from build123d import *

# Parameters (mm, degrees)
F1_DEPTH = 10


with BuildPart() as f1:
    # F0 (on Top) → F1 (new body)
    with BuildSketch(Plane.XY):
        with BuildLine():
            ThreePointArc((2, 4.582576), (4.894532, -1.021548), (0, -5))
            Line((0, -5), (0, -6.00455))
            Line((0, -6.00455), (5, -6.00455))
            Line((5, -6.00455), (5, -16.00455))
            Line((5, -16.00455), (0, -16.00455))
            Line((0, -16.00455), (0, -17.00455))
            Line((0, -17.00455), (6, -17.002946))
            Line((6, -17.002946), (8.996743, -17.002144))
            Line((8.996743, -17.002144), (8.996987, -16.00455))
            Line((8.996987, -16.00455), (9.259669, -14.657077))
            Line((9.259669, -14.657077), (6, -14.657077))
            Line((6, -14.657077), (6, -13.472727))
            Line((6, -13.472727), (9.490384, -13.473582))
            Line((9.490384, -13.473582), (9.731471, -12.236885))
            Line((9.731471, -12.236885), (6, -12.236885))
            Line((6, -12.236885), (6, -11.00455))
            Line((6, -11.00455), (9.971708, -11.00455))
            Line((9.971708, -11.00455), (10.053972, -9.866621))
            Line((10.053972, -9.866621), (6, -9.863548))
            Line((6, -9.863548), (6, -9.04429))
            Line((6, -9.04429), (10.353642, -9.045355))
            Line((10.353642, -9.045355), (10.554617, -8.01442))
            Line((10.554617, -8.01442), (6, -8.01442))
            Line((6, -8.01442), (6, -6.00455))
            Line((6, -6.00455), (10.946429, -6.00455))
            Line((10.946429, -6.00455), (11.140614, -5.008447))
            Line((11.140614, -5.008447), (6, -5.00455))
            Line((6, -5.00455), (3.316625, -5))
            ThreePointArc((3.316625, -5), (3.879995, -4.57664), (4.389841, -4.090146))
            ThreePointArc((4.389841, -4.090146), (4.809454, -3.587359), (5.171773, -3.041836))
            ThreePointArc((5.171773, -3.041836), (5.483753, -2.434842), (5.724784, -1.796345))
            ThreePointArc((5.724784, -1.796345), (5.863661, -1.271801), (5.954582, -0.736856))
            ThreePointArc((5.954582, -0.736856), (5.999496, -0.077783), (5.971684, 0.582233))
            ThreePointArc((5.971684, 0.582233), (5.902156, 1.079145), (5.791354, 1.56851))
            ThreePointArc((5.791354, 1.56851), (4.789612, 3.61381), (3.097802, 5.138446))
            Line((3.097802, 5.138446), (3.097802, 11.138446))
            Line((3.097802, 11.138446), (2, 11.138446))
            Line((2, 11.138446), (2, 4.582576))
        make_face()
        with BuildLine():
            Line((12.501639, 2.997855), (5.791354, 1.56851))
            ThreePointArc((5.791354, 1.56851), (5.902156, 1.079145), (5.971684, 0.582233))
            Line((5.971684, 0.582233), (12.501639, 1.973166))
            Line((12.501639, 1.973166), (12.501639, 2.997855))
        make_face()
        with BuildLine():
            Line((12.116982, 0), (5.954582, -0.736856))
            ThreePointArc((5.954582, -0.736856), (5.863661, -1.271801), (5.724784, -1.796345))
            Line((5.724784, -1.796345), (11.884799, -1.19102))
            Line((11.884799, -1.19102), (12.116982, 0))
        make_face()
        with BuildLine():
            Line((11.523993, -3.041836), (5.171773, -3.041836))
            ThreePointArc((5.171773, -3.041836), (4.809454, -3.587359), (4.389841, -4.090146))
            Line((4.389841, -4.090146), (11.319631, -4.090146))
            Line((11.319631, -4.090146), (11.523993, -3.041836))
        make_face()
        with BuildLine():
            Line((0, -6.00455), (0, -5))
            ThreePointArc((0, -5), (-4.894532, -1.021548), (-2, 4.582576))
            Line((-2, 4.582576), (-2, 11.138446))
            Line((-2, 11.138446), (-3.097802, 11.138446))
            Line((-3.097802, 11.138446), (-3.097802, 5.138446))
            ThreePointArc((-3.097802, 5.138446), (-4.789612, 3.61381), (-5.791354, 1.56851))
            ThreePointArc((-5.791354, 1.56851), (-5.902156, 1.079145), (-5.971684, 0.582233))
            ThreePointArc((-5.971684, 0.582233), (-5.999496, -0.077783), (-5.954582, -0.736856))
            ThreePointArc((-5.954582, -0.736856), (-5.863661, -1.271801), (-5.724784, -1.796345))
            ThreePointArc((-5.724784, -1.796345), (-5.483753, -2.434842), (-5.171773, -3.041836))
            ThreePointArc((-5.171773, -3.041836), (-4.809454, -3.587359), (-4.389841, -4.090146))
            ThreePointArc((-4.389841, -4.090146), (-3.879995, -4.57664), (-3.316625, -5))
            Line((-3.316625, -5), (-6, -5.00455))
            Line((-6, -5.00455), (-11.140614, -5.008447))
            Line((-11.140614, -5.008447), (-10.946429, -6.00455))
            Line((-10.946429, -6.00455), (-6, -6.00455))
            Line((-6, -6.00455), (-6, -8.01442))
            Line((-6, -8.01442), (-10.554617, -8.01442))
            Line((-10.554617, -8.01442), (-10.353642, -9.045355))
            Line((-10.353642, -9.045355), (-6, -9.04429))
            Line((-6, -9.04429), (-6, -9.863548))
            Line((-6, -9.863548), (-10.053972, -9.866621))
            Line((-10.053972, -9.866621), (-9.971708, -11.00455))
            Line((-9.971708, -11.00455), (-6, -11.00455))
            Line((-6, -11.00455), (-6, -12.236885))
            Line((-6, -12.236885), (-9.731471, -12.236885))
            Line((-9.731471, -12.236885), (-9.490384, -13.473582))
            Line((-9.490384, -13.473582), (-6, -13.472727))
            Line((-6, -13.472727), (-6, -14.657077))
            Line((-6, -14.657077), (-9.259669, -14.657077))
            Line((-9.259669, -14.657077), (-8.996987, -16.00455))
            Line((-8.996987, -16.00455), (-8.996743, -17.002144))
            Line((-8.996743, -17.002144), (-6, -17.002946))
            Line((-6, -17.002946), (0, -17.00455))
            Line((0, -17.00455), (0, -16.00455))
            Line((0, -16.00455), (-5, -16.00455))
            Line((-5, -16.00455), (-5, -6.00455))
            Line((-5, -6.00455), (0, -6.00455))
        make_face()
        with BuildLine():
            ThreePointArc((-5.971684, 0.582233), (-5.902156, 1.079145), (-5.791354, 1.56851))
            Line((-5.791354, 1.56851), (-12.501639, 2.997855))
            Line((-12.501639, 2.997855), (-12.501639, 1.973166))
            Line((-12.501639, 1.973166), (-5.971684, 0.582233))
        make_face()
        with BuildLine():
            ThreePointArc((-5.724784, -1.796345), (-5.863661, -1.271801), (-5.954582, -0.736856))
            Line((-5.954582, -0.736856), (-12.116982, 0))
            Line((-12.116982, 0), (-11.884799, -1.19102))
            Line((-11.884799, -1.19102), (-5.724784, -1.796345))
        make_face()
        with BuildLine():
            ThreePointArc((-4.389841, -4.090146), (-4.809454, -3.587359), (-5.171773, -3.041836))
            Line((-5.171773, -3.041836), (-11.523993, -3.041836))
            Line((-11.523993, -3.041836), (-11.319631, -4.090146))
            Line((-11.319631, -4.090146), (-4.389841, -4.090146))
        make_face()
    extrude(amount=F1_DEPTH)


solid = f1.part
For this review, take the finished solid that the model builds, in its own axes (mm). A direction names the side the tool comes from. Round coordinates to 2 decimals unless told otherwise and drop trailing zeros. Write each loop counter-clockwise with the first axis right and the second up, starting at its lowest first coordinate (ties: lowest second). Pieces come first, ordered by that corner, then holes. Notation, with made-up numbers: M 70,25.25 L 115,25.25 A29 cw 115,54.25 Z; hole C 3,58 d3. An arc over 180 degrees is marked long. Write item = value, one per line. Start each with the question number.
(1) We need section B-B (x = 7). Give the number of separate pieces and of enclosed holes in the cut face, then the cut area to 3 significant figures.
(2) We need section A-A (y = 7.75). Give the boundary of the cut face in (x, z), then the cut area to 3 significant figures.
(3) We need section C-C (y = -15). Give the boundary of the cut face in (x, z).
(4) Clearance check with flat-ended pins moving along their axes: pin 1 Ø4 at (x, z) = (-8, 6.5) entering from +Y (3 decimals); pin 2 Ø3 at (y, z) = (-3, 2.5) entering from +X; pin 3 Ø5 at (y, z) = (8, 7) entering from -X; pin 4 Ø1.5 at (x, y) = (-7.5, -7) entering from -Z. State where each tip first meets the part, or that it passes through.
(5) The part is to be moulded in two halves that separate along X. For faces 4 (the face through (6, -7, 5)), 5 (the face through (2.6, 11.138, 4.9)), 6 (the face through (-6, 0, 5)), say which applies: +X half, -X half, draft (parallel to the pull), parting line (faces both ways), or undercut.
(6) For line 1 along X through (y, z) = (-7, 5.5); line 2 along Y through (x, z) = (4.25, 0.5); line 3 along X through (y, z) = (5, 8), list the stretches that pass through material, from the lowest coordinate up.
(7) For faces 1 (the face through (8, -8.014, 5)), 2 (the face through (-9, -6.005, 5)), 3 (the face through (11.42, -3.57, 4.93)), list the 3-axis set-ups (+Z, -Z, +X, -X, +Y, -Y) from which the entire face can be reached by the end or side of a thin tool; tool diameter is ignored.
Results found:
q1.separate_pieces = 8
q1.enclosed_holes = 0
q1.area = 98.8 mm²
q2.outline = M -3.1,0 L -2,0 L -2,10 L -3.1,10 Z; M 2,0 L 3.1,0 L 3.1,10 L 2,10 Z
q2.area = 22.0 mm²
q3.outline = M -9.19,0 L -5,0 L -5,10 L -9.19,10 Z; M 5,0 L 9.19,0 L 9.19,10 L 5,10 Z
q4.pin_1 = 2.465
q4.pin_2 = 11.52
q4.pin_3 = -3.1
q4.pin_4 = through
q5.face_4 = +X half
q5.face_5 = draft
q5.face_6 = undercut
q6.line_1 = -6 to -5, 5 to 6
q6.line_2 = -17 to -16, -6 to -5, -4.24 to -2.63, 2.63 to 4.24
q6.line_3 = -3.32 to -2, 2 to 3.32
q7.face_1 = +Z, -Z, +X
q7.face_2 = +Z, -Z, -X
q7.face_3 = +Z, -Z, +X, -Y
